```python
from build123d import *

# Parameters (mm, degrees)
SKETCH1_W           = 158.4
SKETCH1_H           = 158.4
BOSS_EXTRUDE1_DEPTH = 3
SKETCH2_R           = 2.125
SKETCH2_R_2         = 11
SKETCH2_R_3         = 4
SKETCH2_W           = 43.911972264
SKETCH2_H           = 20
CUT_EXTRUDE3_DEPTH  = 113.045883459
SKETCH3_W           = 20
SKETCH3_H           = 20
CUT_EXTRUDE4_DEPTH  = 113.045883459
FILLET1_R           = 3


with BuildPart() as part:
    # Sketch1 → Boss-Extrude1 (new body)
    with BuildSketch(Plane(origin=(0, 0, 0), x_dir=(1, 0, 0), z_dir=(0, 1, 0))):
        Rectangle(SKETCH1_W, SKETCH1_H)
    extrude(amount=BOSS_EXTRUDE1_DEPTH)

    # Sketch2 → Cut-Extrude3 (cut, through all)
    with BuildSketch(Plane(origin=(0, 3, 0), x_dir=(1, 0, 0), z_dir=(0, 1, 0))):
        with Locations(Location((-69.2, -49.2, 0), (0, 0, 270))):
            Circle(SKETCH2_R)
        with Locations(Location((-69.2, 49.2, 0), (0, 0, 90))):
            Circle(SKETCH2_R)
        with Locations(Location((-49.2, 69.2, 0), (0, 0, 270))):
            Circle(SKETCH2_R)
        with Locations(Location((49.2, 69.2, 0), (0, 0, 90))):
            Circle(SKETCH2_R)
        with Locations(Location((69.2, 49.2, 0), (0, 0, 270))):
            Circle(SKETCH2_R)
        with Locations(Location((69.2, -49.2, 0), (0, 0, 90))):
            Circle(SKETCH2_R)
        with Locations(Location((49.2, -69.2, 0), (0, 0, 270))):
            Circle(SKETCH2_R)
        with Locations(Location((-49.2, -69.2, 0), (0, 0, 90))):
            Circle(SKETCH2_R)
        with Locations(Location((0, 0, 0), (0, 0, 270))):
            Circle(SKETCH2_R_2)
        with Locations(Location((0, 29, 0), (0, 0, 270))):
            Circle(SKETCH2_R)
        with Locations(Location((25.11473671, -14.5, 0), (0, 0, 270))):
            Circle(SKETCH2_R)
        with Locations(Location((-25.11473671, -14.5, 0), (0, 0, 270))):
            Circle(SKETCH2_R)
        with Locations(Location((0, 19.25, 0), (0, 0, 270))):
            Circle(SKETCH2_R_3)
        with Locations((0, -49.2)):
            Rectangle(SKETCH2_W, SKETCH2_H)
    extrude(amount=-CUT_EXTRUDE3_DEPTH, mode=Mode.SUBTRACT)

    # Sketch3 → Cut-Extrude4 (cut, through all)
    with BuildSketch(Plane(origin=(0, 3, 0), x_dir=(1, 0, 0), z_dir=(0, 1, 0))):
        with Locations((69.2, 69.2)):
            Rectangle(SKETCH3_W, SKETCH3_H)
        with Locations((-69.2, 69.2)):
            Rectangle(SKETCH3_W, SKETCH3_H)
        with Locations((69.2, -69.2)):
            Rectangle(SKETCH3_W, SKETCH3_H)
        with Locations((-69.2, -69.2)):
            Rectangle(SKETCH3_W, SKETCH3_H)
    extrude(amount=-CUT_EXTRUDE4_DEPTH, mode=Mode.SUBTRACT)

    # Fillet1
    fillet1_edges = [part.edges().sort_by_distance(p)[0] for p in [
        (21.955986132, 1.5, 39.2),
        (21.955986132, 1.5, 59.2),
        (-21.955986132, 1.5, 59.2),
        (-21.955986132, 1.5, 39.2),
    ]]
    fillet(fillet1_edges, radius=FILLET1_R)


solid = part.part
```
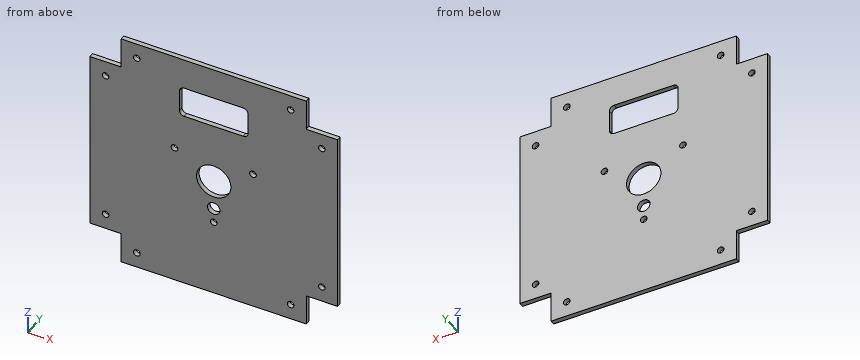
Here's how the part is built. I have some questions about the finished solid (model axes, mm). Give positions to 0.01 mm unless a question says otherwise; leave off trailing zeros. Write each loop counter-clockwise with the first axis right and the second up, starting at its lowest first coordinate (ties: lowest second). Pieces come first, ordered by that corner, then holes. Notation, with made-up numbers: M 25,8.5 L 56,8.5 A30 ccw 56,44.5 Z; hole C 56,-29.5 d4. An arc over 180 degrees is marked long. Put each result on its own line as item: value. Start each with the question number.
Item 1: If we section it at D-D, the plane y = 1.45: Count the separate pieces of the cut face and the enclosed holes in it, then the cut area to 3 significant figures.
Item 2: If we section it at B-B, the plane x = -69.2: Write out the boundary of the cut face in (y, z) (3 decimals), then the cut area to 3 significant figures.
Item 3: Will this pin go through, and if not, where does the flat tip stop? pin 1 (0.9 mm diameter, centred on x = 70.5, y = 2, fed in from +Z).
Item 4: If we section it at A-A, the plane z = 0: Write out the boundary of the cut face in (x, y).
Item 5: I need wall thicknesses on L1, parallel to X at y = 0.9, z = -49.2 (3 decimals); L2, parallel to X at y = 1.75, z = -69.2 (3 decimals); L3, parallel to X at y = 2.3, z = 49.2 (3 decimals). Which ranges of each line are inside material? Lowest first, please. Write a range as from..to.
Item 6: If we section it at C-C, the plane z = 69.2: Write out the boundary of the cut face in (x, y) (3 decimals).
Values:
1. separate pieces: 1
1. enclosed holes: 14
1. area: 22,000 mm²
2. outline: M 0,-59.2 L 3,-59.2 L 3,-51.325 L 0,-51.325 Z; M 0,-47.075 L 3,-47.075 L 3,47.075 L 0,47.075 Z; M 0,51.325 L 3,51.325 L 3,59.2 L 0,59.2 Z
2. area: 330 mm²
3. pin 1: z = 59.2
4. outline: M -79.2,0 L -11,0 L -11,3 L -79.2,3 Z; M 11,0 L 79.2,0 L 79.2,3 L 11,3 Z
5. L1: -79.2..-71.325, -67.075..67.075, 71.325..79.2
5. L2: -59.2..-51.325, -47.075..47.075, 51.325..59.2
5. L3: -79.2..-71.325, -67.075..-21.956, 21.956..67.075, 71.325..79.2
6. outline: M -59.2,0 L -51.325,0 L -51.325,3 L -59.2,3 Z; M -47.075,0 L 47.075,0 L 47.075,3 L -47.075,3 Z; M 51.325,0 L 59.2,0 L 59.2,3 L 51.325,3 Z
